Build history of the part. All positions in model axes, mm. A direction names the side the tool comes from. Round coordinates to 2 decimals unless told otherwise and drop trailing zeros. Loops run counter-clockwise (first coordinate to the right, second up) from the corner with the lowest first, then second, coordinate; pieces in that order, holes last. Notation, with made-up numbers: (65, 5) - (107, 5) arc R17 cw to (107, 30) - close; hole circle Ø9 at (-29.75, 19). An arc over 180 degrees is marked (long way). Put each result on its own line as item: value. Start each with the question number.
from build123d import *

# Parameters (mm, degrees)
SKETCH_W      = 80
SKETCH_H      = 35
PAD_DEPTH     = 120
THICKNESS_T   = -1.5
SKETCH001_W   = 80
SKETCH001_H   = 35
SKETCH001_W_2 = 78.8
SKETCH001_H_2 = 33.8
POCKET_DEPTH  = 10
FILLET001_R   = 1
SKETCH003_W   = 1
SKETCH003_H   = 1.5
PAD002_DEPTH  = 110
FILLET002_R   = 0.89


with BuildPart() as part:
    # Sketch → Pad (new body)
    with BuildSketch(Plane.XY):
        Rectangle(SKETCH_W, SKETCH_H)
    extrude(amount=PAD_DEPTH)

    # Thickness
    thickness_openings = [part.faces().sort_by_distance(p)[0] for p in [
        (0, 0, 120),
    ]]
    offset(amount=THICKNESS_T, openings=thickness_openings)

    # Sketch001 (on Face6 of Thickness) → Pocket (cut)
    with BuildSketch(Plane.XY.offset(120)):
        Rectangle(SKETCH001_W, SKETCH001_H)
        Rectangle(SKETCH001_W_2, SKETCH001_H_2, mode=Mode.SUBTRACT)
    extrude(amount=-POCKET_DEPTH, mode=Mode.SUBTRACT)

    # Fillet001
    fillet001_edges = [part.edges().sort_by_distance(p)[0] for p in [
        (40, -17.5, 55),
        (40, 17.5, 55),
        (-40, -17.5, 55),
        (-40, 17.5, 55),
        (-40, 0, 0),
        (0, -17.5, 0),
        (0, 17.5, 0),
        (40, 0, 0),
    ]]
    fillet(fillet001_edges, radius=FILLET001_R)

    # Sketch003 (on Face28 of Fillet001) → Pad002 (join)
    with BuildSketch(Plane.XY.offset(1.5)):
        with Locations((1.3, 15.25)):
            Rectangle(SKETCH003_W, SKETCH003_H)
        with Locations((-1.2, -15.25)):
            Rectangle(SKETCH003_W, SKETCH003_H)
        with Locations((1.3, -15.25)):
            Rectangle(SKETCH003_W, SKETCH003_H)
        with Locations((-1.2, 15.25)):
            Rectangle(SKETCH003_W, SKETCH003_H)
    extrude(amount=PAD002_DEPTH)

    # Fillet002
    fillet002_edges = [part.edges().sort_by_distance(p)[0] for p in [
        (0, -16.9, 120),
        (39.4, 0, 120),
        (0, 16.9, 120),
        (-39.4, 0, 120),
    ]]
    fillet(fillet002_edges, radius=FILLET002_R)


solid = part.part
Item 1: Which spindle directions (+Z, -Z, +X, -X, +Y, -Y) get a long thin tool onto all of the face, cutting with end or side? Do faces 5 (the flat face through (-1, 16.9, 115)), 6 (the flat face through (38.5, 0, 60)), 7 (the flat face through (39.4, 0, 115)), 8 (the flat face through (-39.4, 0, 115)). Say none if no direction does.
Item 2: Drill centre lines: probe 1 along X at (y, z) = (-3.5, 18); probe 2 along Y at (x, z) = (19, 87); probe 3 along Y at (x, z) = (-27, 113). Where is each one in solid material? Low to high. Write a range as [from, to].
Item 3: Two-plate mould, pull along Y, no slides. Class faces 1 (the flat face through (-1, -16.9, 115)), 2 (the flat face through (-1, 17.5, 55)), 3 (the flat face through (-40, 0, 55)), 4 (the flat face through (-0.5, 16, 59.9)): pulls with the +Y half, pulls with the -Y half, needs draft (parallel to the pull), parting line crosses it, or undercut.
Item 4: Slice it at A-A (z = 21.5). Give the cut face in (x, y).
Item 5: Drop flat-ended pins along their axis: pin 1 Ø7.5 at (y, z) = (8, 116.5) entering from +X; pin 2 Ø0.5 at (x, y) = (-1, 15) entering from +Z; pin 3 Ø10 at (y, z) = (-1, 116) entering from -X. Give the stop position or say it passes through.
Computed values:
1. face 5: +Z, +X, -X, +Y
1. face 6: +Z
1. face 7: +Z, +X, +Y, -Y
1. face 8: +Z, -X, +Y, -Y
2. probe 1: x = [-40, -38.5], [38.5, 40]
2. probe 2: y = [-17.5, -16], [16, 17.5]
2. probe 3: y = [-16.9, -16], [16, 16.9]
3. face 1: pulls with the -Y half
3. face 2: pulls with the +Y half
3. face 3: needs draft
3. face 4: undercut
4. outline: (-40, -16.5) arc R1 ccw to (-39, -17.5) - (39, -17.5) arc R1 ccw to (40, -16.5) - (40, 16.5) arc R1 ccw to (39, 17.5) - (-39, 17.5) arc R1 ccw to (-40, 16.5) - close; hole (-38.5, -16) - (-1.7, -16) - (-1.7, -14.5) - (-0.7, -14.5) - (-0.7, -16) - (0.8, -16) - (0.8, -14.5) - (1.8, -14.5) - (1.8, -16) - (38.5, -16) - (38.5, 16) - (1.8, 16) - (1.8, 14.5) - (0.8, 14.5) - (0.8, 16) - (-0.7, 16) - (-0.7, 14.5) - (-1.7, 14.5) - (-1.7, 16) - (-38.5, 16) - close
5. pin 1: stops at x = 39.4
5. pin 2: stops at z = 111.5
5. pin 3: stops at x = -39.4
